```python
from build123d import *

# Parameters (mm, degrees)
SKETCH1_W           = 45
SKETCH1_H           = 25
BOSS_EXTRUDE1_DEPTH = 10
SKETCH2_R           = 1.75
BOSS_EXTRUDE2_DEPTH = 5
FILLET1_R           = 5
CUT_EXTRUDE1_DEPTH  = 10
SKETCH4_W           = 1
SKETCH4_H           = 20
BOSS_EXTRUDE3_DEPTH = 15
BOSS_EXTRUDE4_DEPTH = 11
CHAMFER1_SIZE       = 5


with BuildPart() as part:
    # Sketch1 → Boss-Extrude1 (new body)
    with BuildSketch(Plane.XY):
        Rectangle(SKETCH1_W, SKETCH1_H)
    extrude(amount=BOSS_EXTRUDE1_DEPTH)

    # Sketch2 → Boss-Extrude2 (add)
    with BuildSketch(Plane(origin=(0, 0, 0), x_dir=(-1, 0, 0), z_dir=(0, 0, -1))):
        Polygon((-30, 20), (-30, -20), (0, -27), (30, -20), (30, 20), (0, 27), align=None)
        with Locations((0, 20)):
            Circle(SKETCH2_R, mode=Mode.SUBTRACT)
        with Locations((0, -20)):
            Circle(SKETCH2_R, mode=Mode.SUBTRACT)
    extrude(amount=BOSS_EXTRUDE2_DEPTH)

    # Fillet1
    fillet1_edges = [part.edges().sort_by_distance(p)[0] for p in [
        (0, -27, -2.5),
        (-30, -20, -2.5),
        (-30, 20, -2.5),
        (0, 27, -2.5),
        (30, 20, -2.5),
        (30, -20, -2.5),
    ]]
    fillet(fillet1_edges, radius=FILLET1_R)

    # Sketch3 → Cut-Extrude1 (cut)
    with BuildSketch(Plane(origin=(0, 0, -5), x_dir=(-1, 0, 0), z_dir=(0, 0, -1))):
        Polygon((5, 10), (5, -10), (15, -10), (20, -5), (20, 5), (15, 10), align=None)
    extrude(amount=-CUT_EXTRUDE1_DEPTH, mode=Mode.SUBTRACT)

    # Sketch4 → Boss-Extrude3 (add)
    with BuildSketch(Plane(origin=(5, 0, 0), x_dir=(0, 0, -1), z_dir=(1, 0, 0))):
        with Locations((5.5, 0)):
            Rectangle(SKETCH4_W, SKETCH4_H)
    extrude(amount=BOSS_EXTRUDE3_DEPTH)

    # Sketch5 → Boss-Extrude4 (add)
    with BuildSketch(Plane(origin=(7, 0, 0), x_dir=(0, 0, -1), z_dir=(1, 0, 0))):
        with BuildLine():
            Line((6, 8), (7.5, 8))
            Line((7.5, 8), (7.5, 0))
            Line((7.5, 0), (11.5, -6.92820323))
            ThreePointArc((11.5, -6.92820323), (8.839548107, -7.923623984), (6, -8))
            Line((6, -8), (6, 8))
        make_face()
    extrude(amount=BOSS_EXTRUDE4_DEPTH)

    # Chamfer1
    chamfer1_edges = [part.edges().sort_by_distance(p)[0] for p in [
        (22.5, -12.5, 5),
        (-22.5, -12.5, 5),
        (-22.5, 12.5, 5),
        (22.5, 12.5, 5),
    ]]
    chamfer(chamfer1_edges, length=CHAMFER1_SIZE)


solid = part.part
```
Geometry check sheet. Reference: the model listing, model coordinates, mm. A direction names the side the tool comes from. Coordinates: 2 decimals unless noted, no trailing zeros. Order: outer loops, then holes, each group sorted by start corner. A loop starts at its lowest first (then second) coordinate and runs counter-clockwise, first axis right, second up. Notation, with made-up numbers: (-1, -37) - (41, -37) arc R29 ccw to (41, -8) - close; hole circle Ø8 at (-9, -35.5). An arc over 180 degrees is marked (long way). Answer as a JSON object with one key per item and string values. Group by question number.
Item 1: Sectioned sample at B-B, the plane z = 3. Record the cut outline in (x, y).
Item 2: Draft check along Y on faces 1 (the face through (-20, 10, 5)), 2 (the face through (18, -2, -8)), 3 (the face through (-28.887, -19.177, -2.535)), 4 (the face through (-12, 0, 5)). Enter one of: +Y half, -Y half, draft (parallel to the pull), parting line (faces both ways), or undercut.
Item 3: Sectioned sample at D-D, the plane z = 8. Record the cut outline in (x, y), and give its area (4 significant figures).
Item 4: Depth check by flat-ended pin: pin 1 Ø0.8 at (x, z) = (14, -5.5) entering from +Y; pin 2 Ø3 at (y, z) = (-1.5, 4.5) entering from +X; pin 3 Ø5 at (x, z) = (-7.5, 6.5) entering from -Y. Enter the tip coordinate at first touch or a pass-through.
Item 5: Tool access check on faces 5 (the face through (12, 8, -7)), 6 (the face through (20, -10, 5)), 7 (the face through (-20, 0, 0)), 8 (the face through (-22.5, 0, 5)). Record the directions out of +Z, -Z, +X, -X, +Y, -Y that give a thin tool (end or side, any length) a straight path to the whole face; none if there is none.
Item 6: Sectioned sample at C-C, the plane y = -19. Record the cut outline in (x, z).
Item 7: Sectioned sample at A-A, the plane x = 0. Record the cut outline in (y, z).
Item 8: Scan lines: probe 1 along X at (y, z) = (-3, 2.75); probe 2 along Z at (x, y) = (-26.5, -20); probe 3 along X at (y, z) = (5.5, 9.25). Record each from-to range of solid material in increasing order.
Resolved:
{
 "1": {"outline": "(-22.5, -7.5) - (-17.5, -12.5) - (17.5, -12.5) - (22.5, -7.5) - (22.5, 7.5) - (17.5, 12.5) - (-17.5, 12.5) - (-22.5, 7.5) - close; hole (-20, -5) - (-15, -10) - (-5, -10) - (-5, 10) - (-15, 10) - (-20, 5) - close"},
 "2": {"face 1": "+Y half", "face 2": "draft", "face 3": "-Y half", "face 4": "undercut"},
 "3": {"outline": "(-22.5, -7.5) - (-17.5, -12.5) - (17.5, -12.5) - (22.5, -7.5) - (22.5, 7.5) - (17.5, 12.5) - (-17.5, 12.5) - (-22.5, 7.5) - close", "area": "1,075 mm^2"},
 "4": {"pin 1": "y = 10", "pin 2": "x = 22.5", "pin 3": "y = -12.5"},
 "5": {"face 5": "-Z, +X, -X, +Y", "face 6": "+Z, +X, -Y", "face 7": "-Z", "face 8": "+Z, -X, +Y, -Y"},
 "6": {"outline": "(-29.02, -5) - (-1.44, -5) - (-1.44, 0) - (-29.02, 0) - close; (1.44, -5) - (29.02, -5) - (29.02, 0) - (1.44, 0) - close"},
 "7": {"outline": "(-26.87, -5) - (-21.75, -5) - (-21.75, 0) - (-26.87, 0) - close; (-18.25, -5) - (18.25, -5) - (18.25, 0) - (12.5, 0) - (12.5, 10) - (-12.5, 10) - (-12.5, 0) - (-18.25, 0) - close; (21.75, -5) - (26.87, -5) - (26.87, 0) - (21.75, 0) - close"},
 "8": {"probe 1": "-22.5 to -20, -5 to 22.5", "probe 2": "-5 to 0", "probe 3": "-22.5 to 22.5"}
}
